from build123d import *

# Parameters (mm, degrees)
BOSS_EXTRUDE1_DEPTH      = 8
BOSS_EXTRUDE1_DEPTH_BACK = 0.001
SKETCH1_W                = 30
SKETCH1_H                = 32
SKETCH3_W                = 1.75
SKETCH3_H                = 8
SKETCH3_W_2              = 1.716544358
CUT_EXTRUDE1_DEPTH       = 35.928498393
SKETCH4_R                = 2.1
CUT_EXTRUDE2_DEPTH       = 6


with BuildPart() as part:
    # Sketch1 → Boss-Extrude1 (new, two sides: drawn at the far end of the back side and taken through both)
    with BuildSketch(Plane.XY.offset(-BOSS_EXTRUDE1_DEPTH_BACK)):
        Rectangle(SKETCH1_W, SKETCH1_H)
    extrude(amount=BOSS_EXTRUDE1_DEPTH + BOSS_EXTRUDE1_DEPTH_BACK)

    # Sketch3 → Cut-Extrude1 (cut, through all)
    with BuildSketch(Plane.ZY.offset(15)):
        with Locations((0.874, 1.75)):
            Rectangle(SKETCH3_W, SKETCH3_H)
        with Locations((0.857272179, -8.249968909)):
            Rectangle(SKETCH3_W_2, SKETCH3_H)
    extrude(amount=-CUT_EXTRUDE1_DEPTH, mode=Mode.SUBTRACT)

    # Sketch4 → Cut-Extrude2 (cut)
    with BuildSketch(Plane(origin=(0, 16, 0), x_dir=(1, 0, 0), z_dir=(0, 1, 0))):
        with Locations(Location((-10.153172438, -4.11086305, 0), (0, 0, 270))):
            Circle(SKETCH4_R)
        with Locations(Location((9.800813668, -4.11086305, 0), (0, 0, 270))):
            Circle(SKETCH4_R)
    extrude(amount=-CUT_EXTRUDE2_DEPTH, mode=Mode.SUBTRACT)


solid = part.part
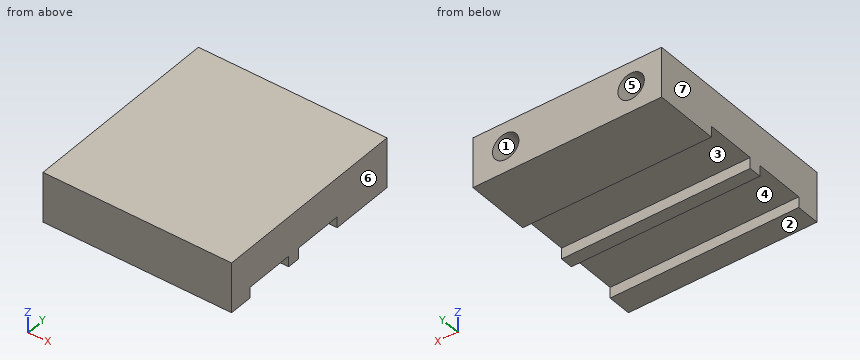
CAD build for the part. Positions are in the model's coordinates, mm. Face numbers are marked on the shaded views. A direction names the side the tool comes from. Round coordinates to 2 decimals unless told otherwise and drop trailing zeros. Write each loop counter-clockwise with the first axis right and the second up, starting at its lowest first coordinate (ties: lowest second). Pieces come first, ordered by that corner, then holes.
(1) Slice it at A-A, the plane x = -4.5. Write the cut outline in (y, z), and give its area (3 significant figures).
(2) Slice it at C-C, the plane y = 5. Write the cut outline in (x, z).
(3) Slice it at B-B, the plane z = 4.5. Write the cut outline in (x, y), and give its area (3 significant figures).
(4) Slice it at D-D, the plane x = 8.5. Write the cut outline in (y, z).
(5) Probe line 1 along X through (y, z) = (11.5, 5.5); line 2 along X through (y, z) = (11.5, 3.25); line 3 along Z through (x, y) = (9.25, 14). List the from-to ranges inside material, lowest first.
(6) 3-axis set-ups, long thin cutter, end or side, ignore diameter. For the marked faces 1, 2 and 3: which of +Z, -Z, +X, -X, +Y, -Y reach the whole face in a straight line?
(7) Mould opens along X. For the marked faces 4, 5, 6 and 7 say: pulls with the +X half, pulls with the -X half, needs draft (parallel to the pull), parting line crosses it, or undercut.
From the geometry:
1. outline: (-16, 0) - (-12.25, 0) - (-12.25, 1.72) - (-4.25, 1.72) - (-4.25, 0) - (-2.25, 0) - (-2.25, 1.75) - (5.75, 1.75) - (5.75, 0) - (16, 0) - (16, 8) - (-16, 8) - close
1. area: 228 mm2
2. outline: (-15, 1.75) - (15, 1.75) - (15, 8) - (-15, 8) - close
3. outline: (-15, -16) - (15, -16) - (15, 16) - (11.86, 16) - (11.86, 10) - (7.74, 10) - (7.74, 16) - (-8.09, 16) - (-8.09, 10) - (-12.22, 10) - (-12.22, 16) - (-15, 16) - close
3. area: 910 mm2
4. outline: (-16, 0) - (-12.25, 0) - (-12.25, 1.72) - (-4.25, 1.72) - (-4.25, 0) - (-2.25, 0) - (-2.25, 1.75) - (5.75, 1.75) - (5.75, 0) - (16, 0) - (16, 2.46) - (10, 2.46) - (10, 5.76) - (16, 5.76) - (16, 8) - (-16, 8) - close
5. line 1: x = -15 to -11.73, -8.58 to 8.23, 11.38 to 15
5. line 2: x = -15 to -12.07, -8.24 to 7.89, 11.72 to 15
5. line 3: z = 0 to 2.08, 6.14 to 8
6. face 1: +Y
6. face 2: -Z, +X, -X, +Y, -Y
6. face 3: -Z, +X, -X
7. face 4: needs draft
7. face 5: undercut
7. face 6: pulls with the +X half
7. face 7: pulls with the -X half
